Source: CAD feature listing. Evaluate the final solid. Frame: model axes, mm. Give positions to 0.01 mm unless a question says otherwise; leave off trailing zeros. Loops run counter-clockwise (first coordinate to the right, second up) from the corner with the lowest first, then second, coordinate; pieces in that order, holes last. Notation, with made-up numbers: M -37.5,20.25 L 4.5,20.25 A24 cw 4.5,30.25 Z; hole C 71,44 d6. An arc over 180 degrees is marked long. Answer in a Markdown table with one row per item.
```python
from build123d import *

# Parameters (mm, degrees)
SKETCH1_W           = 50
SKETCH1_H           = 50
SKETCH1_W_2         = 47
SKETCH1_H_2         = 47
BOSS_EXTRUDE1_DEPTH = 600
SKETCH2_R           = 2.5
CUT_EXTRUDE1_DEPTH  = 59
SKETCH3_R           = 2.5
CUT_EXTRUDE2_DEPTH  = 603.59853966


with BuildPart() as part:
    # Sketch1 → Boss-Extrude1 (new body)
    with BuildSketch(Plane.XY):
        Rectangle(SKETCH1_W, SKETCH1_H)
        Rectangle(SKETCH1_W_2, SKETCH1_H_2, mode=Mode.SUBTRACT)
    extrude(amount=BOSS_EXTRUDE1_DEPTH)

    # Sketch2 → Cut-Extrude1 (cut)
    with BuildSketch(Plane(origin=(25, 0, 0), x_dir=(0, 0, -1), z_dir=(1, 0, 0))):
        with Locations(Location((-300, -15, 0), (0, 0, 90))):
            Circle(SKETCH2_R)
        with Locations(Location((-277, 10, 0), (0, 0, 90))):
            Circle(SKETCH2_R)
        with Locations(Location((-323, 10, 0), (0, 0, 90))):
            Circle(SKETCH2_R)
    extrude(amount=-CUT_EXTRUDE1_DEPTH, mode=Mode.SUBTRACT)

    # Sketch3 → Cut-Extrude2 (cut, through all)
    with BuildSketch(Plane(origin=(0, 25, 0), x_dir=(1, 0, 0), z_dir=(0, 1, 0))):
        with Locations(Location((-10, -40, 0), (0, 0, 270))):
            Circle(SKETCH3_R)
        with Locations(Location((10, -40, 0), (0, 0, 270))):
            Circle(SKETCH3_R)
        with Locations(Location((-10, -60, 0), (0, 0, 270))):
            Circle(SKETCH3_R)
        with Locations(Location((10, -60, 0), (0, 0, 270))):
            Circle(SKETCH3_R)
        with Locations(Location((10, -540, 0), (0, 0, 270))):
            Circle(SKETCH3_R)
        with Locations(Location((-10, -540, 0), (0, 0, 270))):
            Circle(SKETCH3_R)
        with Locations(Location((10, -560, 0), (0, 0, 270))):
            Circle(SKETCH3_R)
        with Locations(Location((-10, -560, 0), (0, 0, 270))):
            Circle(SKETCH3_R)
    extrude(amount=-CUT_EXTRUDE2_DEPTH, mode=Mode.SUBTRACT)


solid = part.part
```
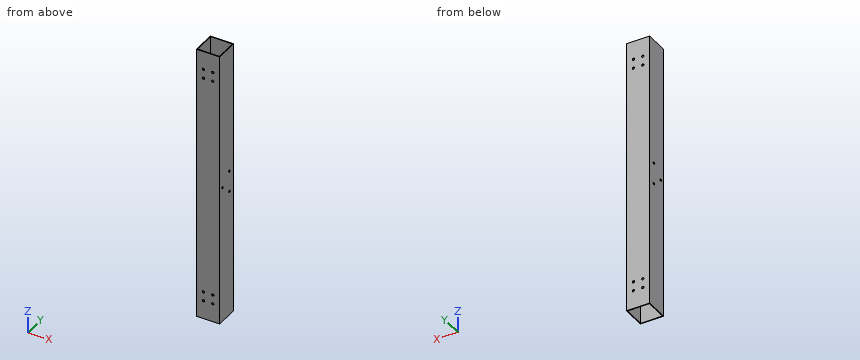
1) Section A-A, the plane y = 2. Return loops of the section in (x, z).
Reply:
| item | result |
|---|---|
| outline | M -25,0 L -23.5,0 L -23.5,600 L -25,600 Z; M 23.5,0 L 25,0 L 25,600 L 23.5,600 Z |
2) Section C-C, the plane z = 246.5. Return loops of the section in (x, y).
Reply:
| item | result |
|---|---|
| outline | M -25,-25 L 25,-25 L 25,25 L -25,25 Z; hole M -23.5,-23.5 L 23.5,-23.5 L 23.5,23.5 L -23.5,23.5 Z |
3) Material intervals for L1, parallel to X at y = -23.9, z = 40; L2, parallel to Y at x = -22.5, z = 421, sorted ascending.
Reply:
| item | result |
|---|---|
| L1 | x = -25 to -12.5, -7.5 to 7.5, 12.5 to 25 |
| L2 | y = -25 to -23.5, 23.5 to 25 |
4) Pin query (flat end, axial travel): pin 1 Ø6 at (y, z) = (-15, 300) entering from -X. Return the tip coordinate at first contact, or that it passes through.
Reply:
| item | result |
|---|---|
| pin 1 | stops at x = -25 |
